from build123d import *

# Parameters (mm, degrees)
F1_DEPTH = 15
F3_DEPTH = 60
F4_SIZE  = 3
F5_R     = 5


with BuildPart() as f1:
    # F0 (on Top) → F1 (new body)
    with BuildSketch(Plane.XY):
        Polygon((-84.375, 42.2187384345), (-78.75, 45.4663336987), (-61.4294919243, 55.4663336987), (-63.9294919243, 59.7964607176), (-72.5897459622, 54.7964607176), (-75.7147459622, 60.2091194913), (-84.375, 55.2091194913), (-81.25, 49.7964607176), (-86.875, 46.5488654534), align=None)
        Polygon((-61.4294919243, 55.4663336987), (-57.0993649054, 57.9663336987), (-59.5993649054, 62.2964607176), (-63.9294919243, 59.7964607176), align=None)
        Polygon((-91.7403810568, 37.9663336987), (-84.375, 42.2187384345), (-86.875, 46.5488654534), (-94.2403810568, 42.2964607176), align=None)
        Polygon((-84.375, 55.2091194913), (-75.7147459622, 60.2091194913), (-85.7147459622, 77.5296275669), (-87.793790014, 76.329290924), (-94.375, 72.5296275669), align=None)
        Polygon((-111.6589653438, 26.4663336987), (-91.7403810568, 37.9663336987), (-94.2403810568, 42.2964607176), (-114.1589653438, 30.7964607176), align=None)
        Polygon((-87.793790014, 76.329290924), (-85.7147459622, 77.5296275669), (-88.8397459622, 82.9422863406), (-75.8493649054, 90.4422863406), (-78.3493115936, 94.7723526968), (-100, 82.2724133595), (-105.625, 79.0248180953), (-103.125, 74.6946910764), (-97.5, 77.9422863406), (-94.375, 72.5296275669), align=None)
        Polygon((-110.4903810568, 70.4422863406), (-103.125, 74.6946910764), (-105.625, 79.0248180953), (-112.9903810568, 74.7724133595), align=None)
        Polygon((-130.4089653438, 58.9422863406), (-110.4903810568, 70.4422863406), (-112.9903810568, 74.7724133595), (-132.9089653438, 63.2724133595), align=None)
    extrude(amount=F1_DEPTH)

    # F2 (on face) → F3 (cut)
    with BuildSketch(Plane(origin=(-39.375, 68.199500548, 0), x_dir=(0.8660254038, 0.5, 0), z_dir=(0.5, -0.8660254038, 0))):
        with BuildLine():
            ThreePointArc((-52.7163336987, 7.5), (-55.4663336987, 10.25), (-58.2163336987, 7.5))
            Line((-58.2163336987, 7.5), (-55.4663336987, 7.5))
            Line((-55.4663336987, 7.5), (-52.7163336987, 7.5))
        make_face()
        with BuildLine():
            Line((-55.4663336987, 7.5), (-58.2163336987, 7.5))
            ThreePointArc((-58.2163336987, 7.5), (-55.4663336987, 4.75), (-52.7163336987, 7.5))
            Line((-52.7163336987, 7.5), (-55.4663336987, 7.5))
        make_face()
        with BuildLine():
            ThreePointArc((-22.8953336987, 7.5), (-25.6453336987, 10.25), (-28.3953336987, 7.5))
            ThreePointArc((-28.3953336987, 7.5), (-25.6453336987, 4.75), (-22.8953336987, 7.5))
        make_face()
    extrude(amount=-F3_DEPTH, mode=Mode.SUBTRACT)

    # F4
    f4_edges = [f1.edges().sort_by_distance(p)[0] for p in [
        (-89.375, 63.869374, 15),
        (-80.714746, 68.869374, 15),
        (-89.375, 63.869374, 0),
        (-80.714746, 68.869374, 0),
    ]]
    chamfer(f4_edges, length=F4_SIZE)

    # F5
    f5_edges = [f1.edges().sort_by_distance(p)[0] for p in [
        (-58.349365, 60.131397, 15),
        (-58.349365, 60.131397, 0),
        (-77.099338, 92.60732, 15),
        (-77.099338, 92.60732, 0),
    ]]
    fillet(f5_edges, radius=F5_R)


solid = f1.part
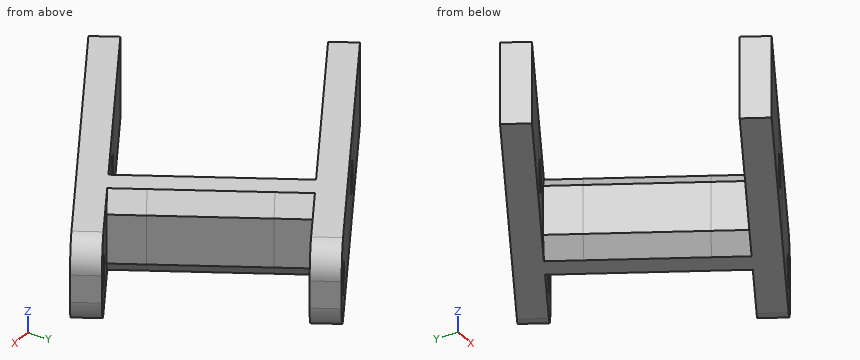
Here's how the part is built. I have some questions about the finished solid (model axes, mm). Give positions to 0.01 mm unless a question says otherwise; leave off trailing zeros. Order: outer loops, then holes, each group sorted by start corner. A loop starts at its lowest first (then second) coordinate and runs counter-clockwise, first axis right, second up. Notation, with made-up numbers: M -24.5,3.25 L 28.5,3.25 A12 cw 28.5,11.25 Z; hole C 24,61.5 d4. An arc over 180 degrees is marked long. Answer as a JSON object with one key per item and string values. Group by question number.
1) I'm going to push flat-ended pins straight in: pin 1 Ø1 at (y, z) = (86.5, 3) entering from -X; pin 2 Ø4 at (x, z) = (-67, 11) entering from +Y; pin 3 Ø1.5 at (x, z) = (-69.5, 13) entering from +Y. Where does each tip first touch, or does it pass through?
2) Suppose I cut it at A-A, the plane y = 67.5. Write out the boundary of the cut face in (x, z), plus the area to 3 significant figures.
3) Please list where these lines run through material, in increasing order: L1, parallel to Y at x = -77, z = 12.5; L2, parallel to Y at x = -101, z = 2.25; L3, parallel to X at y = 67, z = 13.25. Write a range as [from, to].
4) Suppose I cut it at D-D, the plane z = 8.5. Count the separate pieces of the cut face and the enclosed holes in it, plus the area to 3 significant figures.
5) Suppose I cut it at B-B, the plane x = -74. Write out the boundary of the cut face in (y, z), plus the area to 3 significant figures.
Results found:
{
 "1": {"pin 1": "x = -93.54", "pin 2": "y = 59.18", "pin 3": "y = 57.01"},
 "2": {"outline": "M -125.59,0 L -115.59,0 L -115.59,15 L -125.59,15 Z; M -91.47,3 L -88.01,0 L -83.39,0 L -79.92,3 L -79.92,12 L -83.39,15 L -88.01,15 L -91.47,12 Z", "area": "302 mm²"},
 "3": {"L1": "[46.48, 61.44], [89.78, 91.1]", "L2": "[32.62, 38.39], [75.92, 81.7]", "L3": "[-126.45, -116.45], [-89.74, -81.08]"},
 "4": {"separate pieces": "5", "enclosed holes": "0", "area": "853 mm²"},
 "5": {"outline": "M 48.21,0 L 53.98,0 L 53.98,1.37 L 57.24,3 L 57.24,12 L 53.98,13.63 L 53.98,15 L 48.21,15 Z", "area": "121 mm²"}
}
